For this review, take the finished solid that the model builds, in its own axes (mm). A direction names the side the tool comes from. Give positions to 0.01 mm unless a question says otherwise; leave off trailing zeros. Write each loop counter-clockwise with the first axis right and the second up, starting at its lowest first coordinate (ties: lowest second). Pieces come first, ordered by that corner, then holes. Notation, with made-up numbers: M -19.75,59.5 L 1.25,59.5 A23 ccw 1.25,97.5 Z; hole C -34.5,32.5 d11. An arc over 180 degrees is marked long. Use one line per item in the form item = value. Start each with the question number.
Q1. Consider section B-B on y = -79. Write out the cut boundary in (x, z), and give its area (3 significant figures).
Q2. Tool access review of faces 1 (the flat face through (65, 8, 9)), 2 (the flat face through (61, -68, 44.1)), 3 (the flat face through (60, -63, 29.1)), 4 (the flat face through (48, -54.158, 51)): name each direction out of +Z, -Z, +X, -X, +Y, -Y from which nothing blocks a thin tool from reaching the whole face with its end or side.
Q3. Consider section D-D on x = 32. Write out the cut boundary in (y, z), and give its area (3 significant figures).
Q4. Clearance check with flat-ended pins moving along their axes: pin 1 Ø10 at (x, z) = (37.5, 19) entering from -Y; pin 2 Ø1 at (x, y) = (27, -45.5) entering from -Z; pin 3 Ø7.5 at (y, z) = (-67.5, 38) entering from +X. State where each tip first meets the part, or that it passes through.
Q5. Consider section A-A on x = 59.5. Write out the cut boundary in (y, z).
Q6. Consider section C-C on y = -3.5. Write out the cut boundary in (x, z), and give its area (3 significant figures).
Q7. For probe 1 along Y at (x, z) = (55, 41); probe 2 along Z at (x, y) = (63, -1); probe 3 along Y at (x, z) = (49.5, 11), list the stretches that pass through material, from the lowest coordinate up. Write a range as [from, to].
Q8. Mouldability with a two-part tool opening along Y and no side actions: class faces 5 (the flat face through (65, -69, 36)), 6 (the flat face through (26, -60, 31)), 7 (the flat face through (46, -9, 44.1)), 8 (the flat face through (36, -13.1, 22)) as released by +Y, released by -Y, zero draft, split by the parting line, or undercut.
```python
from build123d import *

# Parameters (mm, degrees)
SKETCH_1_W          = 50
SKETCH_1_H          = 60
EXTRUDE_1_DEPTH     = 44.1
SKETCH_2_W          = 113
SKETCH_2_H          = 33.8
CUT_EXTRUDE_1_DEPTH = 120.456310005
CUT_EXTRUDE_2_DEPTH = 10
EXTRUDE_2_DEPTH     = 14
SKETCH_5_W          = 67
SKETCH_5_H          = 60
EXTRUDE_3_DEPTH     = 5


with BuildPart() as part:
    # 草图1 → 凸台-拉伸1 (new body)
    with BuildSketch(Plane.XY):
        with Locations((25, -30)):
            Rectangle(SKETCH_1_W, SKETCH_1_H)
        Polygon((50, 0), (50, -30), (65, -30), (65, 30), align=None)
        Polygon((65, -30), (50, -30), (50, -60), (65, -90), align=None)
    extrude(amount=EXTRUDE_1_DEPTH)

    # 草图2 → 切除-拉伸1 (cut, through all)
    with BuildSketch(Plane.XY.offset(44.1)):
        with Locations((65, -30)):
            Rectangle(SKETCH_2_W, SKETCH_2_H)
    extrude(amount=-CUT_EXTRUDE_1_DEPTH, mode=Mode.SUBTRACT)

    # 草图3 → 切除-拉伸2 (cut)
    with BuildSketch(Plane(origin=(65, 0, 0), x_dir=(0, 0, -1), z_dir=(1, 0, 0))):
        Polygon((-19.1, -38.027210884), (-28.26075, -13.1), (-29.1, -13.1), (-29.1, -90), (-19.1, -90), align=None)
        Polygon((-29.1, 30), (-29.1, -10.816326531), (-28.26075, -13.1), (-19.1, -13.1), (-19.1, 30), align=None)
    extrude(amount=-CUT_EXTRUDE_2_DEPTH, mode=Mode.SUBTRACT)

    # 草图4 → 凸台-拉伸2 (add)
    with BuildSketch(Plane.XY.offset(44.1)):
        Polygon((0, 0), (0, -60), (67, -60), (67, -54.158468487), (28.5, -54.158468487), (28.5, -4.836475325), (67, -4.836475325), (67, 0), align=None)
    extrude(amount=EXTRUDE_2_DEPTH)

    # 草图5 → 凸台-拉伸3 (add)
    with BuildSketch(Plane.XY.offset(58.1)):
        with Locations((33.5, -30)):
            Rectangle(SKETCH_5_W, SKETCH_5_H)
    extrude(amount=EXTRUDE_3_DEPTH)


solid = part.part
```
Working result:
q1.outline = M 59.5,0 L 65,0 L 65,19.1 L 59.5,19.1 Z; M 59.5,29.1 L 65,29.1 L 65,44.1 L 59.5,44.1 Z
q1.area = 188 mm²
q2.face_1 = -Z, +X, +Y, -Y
q2.face_2 = +Z, +X, -X, -Y
q2.face_3 = +X, -Y
q2.face_4 = +X
q3.outline = M -60,0 L -46.9,0 L -46.9,44.1 L -54.16,44.1 L -54.16,58.1 L -4.84,58.1 L -4.84,44.1 L -13.1,44.1 L -13.1,0 L 0,0 L 0,63.1 L -60,63.1 Z
q3.area = 1,600 mm²
q4.pin_1 = -60
q4.pin_2 = 44.1
q4.pin_3 = 65
q5.outline = M -79,0 L -46.9,0 L -46.9,19.1 L -79,19.1 Z; M -79,29.1 L -46.9,29.1 L -46.9,44.1 L -54.16,44.1 L -54.16,58.1 L -4.84,58.1 L -4.84,44.1 L -13.1,44.1 L -13.1,28.26 L -10.82,29.1 L 19,29.1 L 19,44.1 L 0,44.1 L 0,63.1 L -60,63.1 L -60,44.1 L -79,44.1 Z; M -13.1,0 L 19,0 L 19,19.1 L -13.1,19.1 Z
q6.outline = M 0,0 L 65,0 L 65,19.1 L 55,19.1 L 55,29.1 L 65,29.1 L 65,44.1 L 67,44.1 L 67,63.1 L 0,63.1 Z
q6.area = 4,040 mm²
q7.probe_1 = [-70, -46.9], [-13.1, 10]
q7.probe_2 = [0, 19.1], [29.1, 63.1]
q7.probe_3 = [-60, -46.9], [-13.1, 0]
q8.face_5 = zero draft
q8.face_6 = released by -Y
q8.face_7 = undercut
q8.face_8 = undercut
